Here's the drawing with two shaded views (mm, measured from the low corner). I have some questions. Give positions to 0.01 mm unless a question says otherwise; leave off trailing zeros. Loops run counter-clockwise (first coordinate to the right, second up) from the corner with the lowest first, then second, coordinate; pieces in that order, holes last. Notation, with made-up numbers: (86, 83) -> (137, 83) arc R24 cw to (137, 109) -> close; hole circle Ø11 at (-1, -32.75). An arc over 180 degrees is marked (long way). Put each result on its own line as item: value.
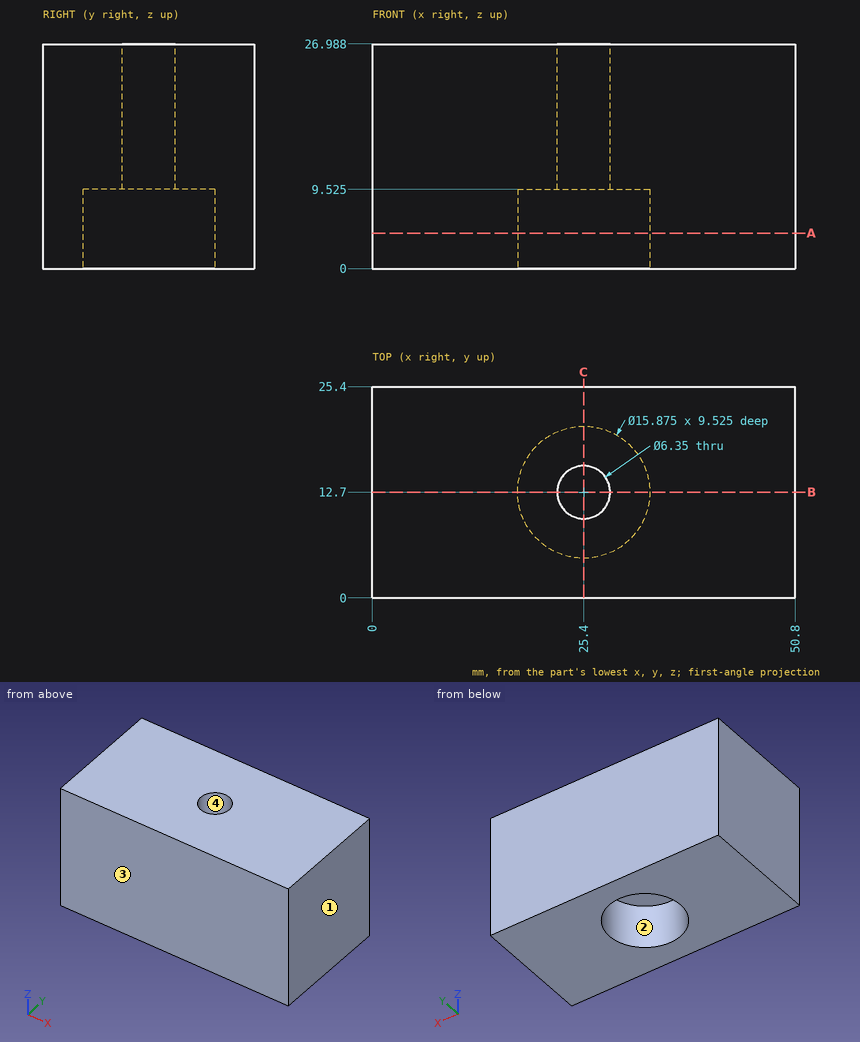
1. Thinking about a two-plate mould opening in X: for the marked faces 1, 2, 3 and 4, which applies, pulls with the +X half, pulls with the -X half, needs draft (parallel to the pull), parting line crosses it, or undercut?
Recorded:
face 1: pulls with the +X half
face 2: undercut
face 3: needs draft
face 4: undercut
2. I need wall thicknesses on line 1 (Y direction, x = 25.4, z = 23.25) (1 decimal); line 2 (Y direction, x = 25.4, z = 3.5); line 3 (X direction, y = 9.25, z = 4.5). Which ranges of each line are inside material? Lowest first, please.
Recorded:
line 1: y = 0 to 9.5, 15.9 to 25.4
line 2: y = 0 to 4.76, 20.64 to 25.4
line 3: x = 0 to 18.25, 32.55 to 50.8
3. If we section it at C-C (x = 25.4): List the corners of the cut face in (y, z) for me (1 decimal).
Recorded:
outline: (0, 0) -> (4.8, 0) -> (4.8, 9.5) -> (9.5, 9.5) -> (9.5, 27) -> (0, 27) -> close; (15.9, 9.5) -> (20.6, 9.5) -> (20.6, 0) -> (25.4, 0) -> (25.4, 27) -> (15.9, 27) -> close
4. If we section it at B-B (y = 12.7): List the corners of the cut face in (x, z) for me (1 decimal), then the cut area to 3 significant figures.
Recorded:
outline: (0, 0) -> (17.5, 0) -> (17.5, 9.5) -> (22.2, 9.5) -> (22.2, 27) -> (0, 27) -> close; (28.6, 9.5) -> (33.3, 9.5) -> (33.3, 0) -> (50.8, 0) -> (50.8, 27) -> (28.6, 27) -> close
area: 1,110 mm^2
5. I'm going to push flat-ended pins straight in: pin 1 (5 mm diameter, centred on y = 7.5, z = 8, fed in from -X); pin 2 (8 mm diameter, centred on x = 25.5, y = 13.5, fed in from -Z) (1 decimal). Where does each tip first touch, or does it pass through?
Recorded:
pin 1: stops at x = 0
pin 2: stops at z = 9.5
6. If we section it at A-A (z = 4.25): List the corners of the cut face in (x, y) for me (1 decimal), then the cut area to 3 significant figures.
Recorded:
outline: (0, 0) -> (50.8, 0) -> (50.8, 25.4) -> (0, 25.4) -> close; hole circle Ø15.9 at (25.4, 12.7)
area: 1,090 mm^2
